from build123d import *

# Parameters (mm, degrees)
F0_W         = 381
F0_H         = 101.6
F1_DEPTH     = 127
F2_W         = 369.2652
F2_H         = 115.2652
F3_DEPTH     = 92.456
F4_W         = 7.62
F4_H         = 115.2652
F5_DEPTH     = 92.202
F6_W         = 5.08
F6_H         = 115.2652
F7_DEPTH     = 91.948
F8_R         = 5.08
F9_T1_DEPTH  = 383.54
F9_T3_DEPTH  = 109.22
F9_T5_DEPTH  = 401.32
F9_T7_DEPTH  = 129.54
F9_S11_W     = 5.1816
F9_S11_H     = 5.1816
F9_T12_DEPTH = 5.1816


# Not quite as in the source:
# - a fillet or chamfer that OpenCascade refuses, or shapes differently, is made with other operations: its cross-section is extruded or revolved along the edge and cut away or added


with BuildPart() as f1:
    # F0 (on Top) → F1 (new body)
    with BuildSketch(Plane.XY):
        Rectangle(F0_W, F0_H)
    extrude(amount=F1_DEPTH)

    # F2 (on face) → F3 (cut)
    with BuildSketch(Plane.XZ.offset(50.8)):
        with Locations((0, 63.5)):
            Rectangle(F2_W, F2_H)
    extrude(amount=-F3_DEPTH, mode=Mode.SUBTRACT)

    # F4 (on face) → F5 (join)
    with BuildSketch(Plane.XZ.offset(-41.656)):
        with Locations((-61.4426, 63.5)):
            Rectangle(F4_W, F4_H)
    extrude(amount=F5_DEPTH)

    # F6 (on face) → F7 (join)
    with BuildSketch(Plane.XZ.offset(-41.656)):
        with Locations((60.1726, 63.5)):
            Rectangle(F6_W, F6_H)
    extrude(amount=F7_DEPTH)

    # F8
    f8_edges = [f1.edges().sort_by_distance(p)[0] for p in [
        (0, 50.8, 0),
        (-190.5, 0, 0),
        (0, -50.8, 0),
        (190.5, 0, 0),
        (-190.5, 50.8, 63.5),
        (-190.5, -50.8, 63.5),
        (-190.5, 0, 127),
    ]]
    fillet(f8_edges, radius=F8_R)

    # F9: fillet of radius 5.08 on 7 edges, made by hand

    # F9_s2 → F9_t1 (cut)
    with BuildSketch(Plane.YZ.offset(-198.12)):
        with BuildLine():
            ThreePointArc((50.8, 121.92), (49.3121024484, 125.5121024484), (45.72, 127))
            Line((45.72, 127), (50.8, 127))
            Line((50.8, 127), (50.8, 121.92))
        make_face()
    extrude(amount=F9_T1_DEPTH, mode=Mode.SUBTRACT)

    # F9_s4 → F9_t3 (cut)
    with BuildSketch(Plane.XZ.offset(-45.72)):
        with BuildLine():
            ThreePointArc((190.5, 121.92), (189.0121024484, 125.5121024484), (185.42, 127))
            Line((185.42, 127), (190.5, 127))
            Line((190.5, 127), (190.5, 121.92))
        make_face()
    extrude(amount=F9_T3_DEPTH, mode=Mode.SUBTRACT)

    # F9_s6 → F9_t5 (cut)
    with BuildSketch(Plane.YZ.offset(-198.12)):
        with BuildLine():
            ThreePointArc((-45.72, 127), (-49.3121024484, 125.5121024484), (-50.8, 121.92))
            Line((-50.8, 121.92), (-50.8, 127))
            Line((-50.8, 127), (-45.72, 127))
        make_face()
    extrude(amount=F9_T5_DEPTH, mode=Mode.SUBTRACT)

    # F9_s8 → F9_t7 (cut)
    with BuildSketch(Plane.XY.offset(-7.62)):
        with BuildLine():
            ThreePointArc((185.42, 50.8), (189.0121024484, 49.3121024484), (190.5, 45.72))
            Line((190.5, 45.72), (190.5, 50.8))
            Line((190.5, 50.8), (185.42, 50.8))
        make_face()
    extrude(amount=F9_T7_DEPTH, mode=Mode.SUBTRACT)


with BuildPart() as f9_tool10:
    # F9_s11 → F9_t12 (new body)
    with BuildSketch(Plane.XZ.offset(-45.72)):
        with Locations((188.0108, 124.5108)):
            Rectangle(F9_S11_W, F9_S11_H)
    extrude(amount=-F9_T12_DEPTH)

    # F9_s13 → F9_t14 (revolve, cut)
    with BuildSketch(Plane(origin=(185.42, 45.72, 121.92), x_dir=(-0.7071067812, 0, -0.7071067812), z_dir=(0.7071067812, 0, -0.7071067812))):
        with BuildLine():
            ThreePointArc((0, -5.08), (5.08, 0), (0, 5.08))
            Line((0, 5.08), (0, -5.08))
        make_face()
    revolve(axis=Axis((185.42, 45.72, 121.92), (0, 1, 0)), mode=Mode.SUBTRACT)


with BuildPart() as f1_1:
    add(f1.part)

    # F9_t9: cut F9_tool10
    add(f9_tool10.part, mode=Mode.SUBTRACT)


solid = f1_1.part
Check sheet for the modelled part. Datum: model origin and axes. Units: mm. A direction names the side the tool comes from. Give positions to 0.01 mm unless a question says otherwise; leave off trailing zeros. Write each loop counter-clockwise with the first axis right and the second up, starting at its lowest first coordinate (ties: lowest second). Pieces come first, ordered by that corner, then holes. Notation, with made-up numbers: (32, 3.25) -> (82, 3.25) arc R31 cw to (82, 28.25) -> close; hole circle Ø5 at (66, -14). An arc over 180 degrees is marked (long way). Write item = value, one per line.
Item 1: Release check for a two-part mould opening along X. For faces 3 (the flat face through (57.633, -4, 63)), 4 (the flat face through (190.5, -3, 63)), 5 (the flat face through (-3, 50.8, 63)) record: +X half, -X half, draft (parallel to the pull), parting line (faces both ways), or undercut.
Output:
face_3 = undercut
face_4 = +X half
face_5 = draft
Item 2: Scan lines: probe 1 along X at (y, z) = (-17.5, 99); probe 2 along Z at (x, y) = (54.5, 30); probe 3 along Y at (x, z) = (166, 16.5). Record each from-to range of solid material in increasing order. Write a range as from..to.
Output:
probe_1 = -190.5..-184.63, -65.25..-57.63, 57.63..62.71, 184.63..190.5
probe_2 = 0..5.87, 121.13..127
probe_3 = 41.66..50.8
Item 3: Gauge pin test, flat ends, axial feed: pin 1 (6 mm diameter, centred on x = -130.5, z = 106, fed in from -Y); pin 2 (1.5 mm diameter, centred on x = 60.5, z = 47, fed in from -Y); pin 3 (2.5 mm diameter, centred on x = -60, z = 84, fed in from -Y). Record the tip position at first contact, or that the pin passes through.
Output:
pin_1 = 41.66
pin_2 = -50.29
pin_3 = -50.55
Item 4: Sectioned sample at B-B on x = -99. Record the boundary of the cut face in (y, z).
Output:
outline = (-50.8, 5.08) arc R5.08 ccw to (-45.72, 0) -> (45.72, 0) arc R5.08 ccw to (50.8, 5.08) -> (50.8, 121.92) arc R5.08 ccw to (45.72, 127) -> (-45.72, 127) arc R5.08 ccw to (-50.8, 121.92) -> (-50.8, 121.13) -> (41.66, 121.13) -> (41.66, 5.87) -> (-50.8, 5.87) -> close
Item 5: Sectioned sample at A-A on y = 8. Record the boundary of the cut face in (x, z).
Output:
outline = (-190.5, 5.08) arc R5.08 ccw to (-185.42, 0) -> (185.42, 0) arc R5.08 ccw to (190.5, 5.08) -> (190.5, 121.92) arc R5.08 ccw to (185.42, 127) -> (-185.42, 127) arc R5.08 ccw to (-190.5, 121.92) -> close; hole (-184.63, 5.87) -> (-65.25, 5.87) -> (-65.25, 121.13) -> (-184.63, 121.13) -> close; hole (-57.63, 5.87) -> (57.63, 5.87) -> (57.63, 121.13) -> (-57.63, 121.13) -> close; hole (62.71, 5.87) -> (184.63, 5.87) -> (184.63, 121.13) -> (62.71, 121.13) -> close
Item 6: Sectioned sample at C-C on z = 81. Record the boundary of the cut face in (x, y), and give its area (3 significant figures).
Output:
outline = (-190.5, -45.72) arc R5.08 ccw to (-185.42, -50.8) -> (-184.63, -50.8) -> (-184.63, 41.66) -> (-65.25, 41.66) -> (-65.25, -50.55) -> (-57.63, -50.55) -> (-57.63, 41.66) -> (57.63, 41.66) -> (57.63, -50.29) -> (62.71, -50.29) -> (62.71, 41.66) -> (184.63, 41.66) -> (184.63, -50.8) -> (190.5, -50.8) -> (190.5, 45.72) arc R5.08 ccw to (185.42, 50.8) -> (-185.42, 50.8) arc R5.08 ccw to (-190.5, 45.72) -> close
area = 5,720 mm^2
Item 7: Tool access check on faces 1 (the flat face through (-3, 1, 0)), 2 (the flat face through (-1, 41.656, 64)). Record the directions out of +Z, -Z, +X, -X, +Y, -Y that give a thin tool (end or side, any length) a straight path to the whole face; none if there is none.
Output:
face_1 = -Z, +X, -X, +Y, -Y
face_2 = -Y
